```python
from build123d import *

# Parameters (mm, degrees)
SKETCH1_W               = 120
SKETCH1_H               = 85
BOSS_EXTRUDE1_DEPTH     = 17.5
SKETCH2_R               = 6.25
CUT_EXTRUDE1_DEPTH      = 34
SKETCH5_R               = 4
CUT_EXTRUDE4_DEPTH      = 82.432487375
FILLET1_R               = 5
SKETCH3_W               = 104.211367546
SKETCH3_H               = 27
CUT_EXTRUDE2_DEPTH      = 106.50473923
SKETCH4_W               = 69.558922102
SKETCH4_H               = 27
CUT_EXTRUDE3_DEPTH      = 129.500972759
SKETCH6_W               = 4
SKETCH6_H               = 4
BOSS_EXTRUDE2_DEPTH     = 35
CHAMFER1_SIZE           = 1
CHAMFER3_SIZE           = 1
CUT_EXTRUDE8_DEPTH      = 76.581082289
CUT_EXTRUDE8_DEPTH_BACK = 13.5
SKETCH10_W              = 127.378136422
SKETCH10_H              = 96.398058909
SKETCH11_W              = 4
SKETCH11_H              = 4
CUT_EXTRUDE9_DEPTH      = 82.432487375


with BuildPart() as part:
    # Sketch1 → Boss-Extrude1 (new, symmetric)
    with BuildSketch(Plane(origin=(0, 0, 0), x_dir=(1, 0, 0), z_dir=(0, 1, 0))):
        Rectangle(SKETCH1_W, SKETCH1_H)
    extrude(amount=BOSS_EXTRUDE1_DEPTH, both=True)

    # Sketch2 → Cut-Extrude1 (cut)
    with BuildSketch(Plane(origin=(0, 17.5, 0), x_dir=(1, 0, 0), z_dir=(0, 1, 0))):
        with Locations(Location((-45.56575, 27, 0), (0, 0, 270))):
            Circle(SKETCH2_R)
        with Locations(Location((-27.33945, 27, 0), (0, 0, 270))):
            Circle(SKETCH2_R)
        with Locations(Location((-9.11315, 27, 0), (0, 0, 270))):
            Circle(SKETCH2_R)
        with Locations(Location((9.11315, 27, 0), (0, 0, 270))):
            Circle(SKETCH2_R)
        with Locations(Location((27.33945, 27, 0), (0, 0, 270))):
            Circle(SKETCH2_R)
        with Locations(Location((45.56575, 27, 0), (0, 0, 270))):
            Circle(SKETCH2_R)
        with Locations(Location((-27.33945, 9, 0), (0, 0, 270))):
            Circle(SKETCH2_R)
        with Locations(Location((-9.11315, 9, 0), (0, 0, 270))):
            Circle(SKETCH2_R)
        with Locations(Location((9.11315, 9, 0), (0, 0, 270))):
            Circle(SKETCH2_R)
        with Locations(Location((27.33945, 9, 0), (0, 0, 270))):
            Circle(SKETCH2_R)
        with Locations(Location((45.56575, 9, 0), (0, 0, 270))):
            Circle(SKETCH2_R)
        with Locations(Location((-27.33945, -9, 0), (0, 0, 270))):
            Circle(SKETCH2_R)
        with Locations(Location((-9.11315, -9, 0), (0, 0, 270))):
            Circle(SKETCH2_R)
        with Locations(Location((9.11315, -9, 0), (0, 0, 270))):
            Circle(SKETCH2_R)
        with Locations(Location((27.33945, -9, 0), (0, 0, 270))):
            Circle(SKETCH2_R)
        with Locations(Location((45.56575, -9, 0), (0, 0, 270))):
            Circle(SKETCH2_R)
        with Locations(Location((-27.33945, -27, 0), (0, 0, 270))):
            Circle(SKETCH2_R)
        with Locations(Location((-9.11315, -27, 0), (0, 0, 270))):
            Circle(SKETCH2_R)
        with Locations(Location((9.11315, -27, 0), (0, 0, 270))):
            Circle(SKETCH2_R)
        with Locations(Location((27.33945, -27, 0), (0, 0, 270))):
            Circle(SKETCH2_R)
        with Locations(Location((45.56575, -27, 0), (0, 0, 270))):
            Circle(SKETCH2_R)
        with Locations(Location((-45.56575, 9, 0), (0, 0, 270))):
            Circle(SKETCH2_R)
        with Locations(Location((-45.56575, -9, 0), (0, 0, 270))):
            Circle(SKETCH2_R)
        with Locations(Location((-45.56575, -27, 0), (0, 0, 270))):
            Circle(SKETCH2_R)
    extrude(amount=-CUT_EXTRUDE1_DEPTH, mode=Mode.SUBTRACT)

    # Sketch5 → Cut-Extrude4 (cut, through all)
    with BuildSketch(Plane(origin=(0, 17.5, 0), x_dir=(1, 0, 0), z_dir=(0, 1, 0))):
        with Locations(Location((-45.56575, 27, 0), (0, 0, 270))):
            Circle(SKETCH5_R)
        with Locations(Location((-27.336055, 27, 0), (0, 0, 270))):
            Circle(SKETCH5_R)
        with Locations(Location((-9.10636, 27, 0), (0, 0, 270))):
            Circle(SKETCH5_R)
        with Locations(Location((9.123335, 27, 0), (0, 0, 270))):
            Circle(SKETCH5_R)
        with Locations(Location((27.35303, 27, 0), (0, 0, 270))):
            Circle(SKETCH5_R)
        with Locations(Location((45.582725, 27, 0), (0, 0, 270))):
            Circle(SKETCH5_R)
        with Locations(Location((-27.336055, 9, 0), (0, 0, 270))):
            Circle(SKETCH5_R)
        with Locations(Location((-9.10636, 9, 0), (0, 0, 270))):
            Circle(SKETCH5_R)
        with Locations(Location((9.123335, 9, 0), (0, 0, 270))):
            Circle(SKETCH5_R)
        with Locations(Location((27.35303, 9, 0), (0, 0, 270))):
            Circle(SKETCH5_R)
        with Locations(Location((45.582725, 9, 0), (0, 0, 270))):
            Circle(SKETCH5_R)
        with Locations(Location((-27.336055, -9, 0), (0, 0, 270))):
            Circle(SKETCH5_R)
        with Locations(Location((-9.10636, -9, 0), (0, 0, 270))):
            Circle(SKETCH5_R)
        with Locations(Location((9.123335, -9, 0), (0, 0, 270))):
            Circle(SKETCH5_R)
        with Locations(Location((27.35303, -9, 0), (0, 0, 270))):
            Circle(SKETCH5_R)
        with Locations(Location((45.582725, -9, 0), (0, 0, 270))):
            Circle(SKETCH5_R)
        with Locations(Location((-27.336055, -27, 0), (0, 0, 270))):
            Circle(SKETCH5_R)
        with Locations(Location((-9.10636, -27, 0), (0, 0, 270))):
            Circle(SKETCH5_R)
        with Locations(Location((9.123335, -27, 0), (0, 0, 270))):
            Circle(SKETCH5_R)
        with Locations(Location((27.35303, -27, 0), (0, 0, 270))):
            Circle(SKETCH5_R)
        with Locations(Location((45.582725, -27, 0), (0, 0, 270))):
            Circle(SKETCH5_R)
        with Locations(Location((-45.56575, 9, 0), (0, 0, 270))):
            Circle(SKETCH5_R)
        with Locations(Location((-45.56575, -9, 0), (0, 0, 270))):
            Circle(SKETCH5_R)
        with Locations(Location((-45.56575, -27, 0), (0, 0, 270))):
            Circle(SKETCH5_R)
    extrude(amount=-CUT_EXTRUDE4_DEPTH, mode=Mode.SUBTRACT)

    # Fillet1
    fillet1_edges = [part.edges().sort_by_distance(p)[0] for p in [
        (60, 0, 42.5),
        (-60, 0, 42.5),
        (-60, 0, -42.5),
        (60, 0, -42.5),
    ]]
    fillet(fillet1_edges, radius=FILLET1_R)

    # Sketch3 → Cut-Extrude2 (cut, through all)
    with BuildSketch(Plane(origin=(0, 0, -42.5), x_dir=(-1, 0, 0), z_dir=(0, 0, -1))):
        Rectangle(SKETCH3_W, SKETCH3_H)
    extrude(amount=-CUT_EXTRUDE2_DEPTH, mode=Mode.SUBTRACT)

    # Sketch4 → Cut-Extrude3 (cut, through all)
    with BuildSketch(Plane(origin=(60, 0, 0), x_dir=(0, 0, -1), z_dir=(1, 0, 0))):
        Rectangle(SKETCH4_W, SKETCH4_H)
    extrude(amount=-CUT_EXTRUDE3_DEPTH, mode=Mode.SUBTRACT)

    # Sketch6 → Boss-Extrude2 (add)
    with BuildSketch(Plane(origin=(0, 17.5, 0), x_dir=(1, 0, 0), z_dir=(0, 1, 0))):
        Rectangle(SKETCH6_W, SKETCH6_H)
    extrude(amount=-BOSS_EXTRUDE2_DEPTH)

    # Chamfer1
    chamfer1_edges = [part.edges().sort_by_distance(p)[0] for p in [
        (0, 13.5, -2),
        (-2, 13.5, 0),
        (0, 13.5, 2),
        (2, 13.5, 0),
        (2, -13.5, 0),
        (0, -13.5, 2),
        (-2, -13.5, 0),
        (0, -13.5, -2),
    ]]
    chamfer(chamfer1_edges, length=CHAMFER1_SIZE)

    # Chamfer3
    chamfer3_edges = [part.edges().sort_by_distance(p)[0] for p in [
        (-45.56575, 17.5, -33.25),
        (-27.33945, 17.5, -33.25),
        (-9.11315, 17.5, -33.25),
        (9.11315, 17.5, -33.25),
        (27.33945, 17.5, -33.25),
        (45.56575, 17.5, -33.25),
        (-27.33945, 17.5, -15.25),
        (-9.11315, 17.5, -15.25),
        (9.11315, 17.5, -15.25),
        (27.33945, 17.5, -15.25),
        (45.56575, 17.5, -15.25),
        (-27.33945, 17.5, 2.75),
        (-9.11315, 17.5, 2.75),
        (9.11315, 17.5, 2.75),
        (27.33945, 17.5, 2.75),
        (45.56575, 17.5, 2.75),
        (-27.33945, 17.5, 20.75),
        (-9.11315, 17.5, 20.75),
        (9.11315, 17.5, 20.75),
        (27.33945, 17.5, 20.75),
        (45.56575, 17.5, 20.75),
        (-45.56575, 17.5, -15.25),
        (-45.56575, 17.5, 2.75),
        (-45.56575, 17.5, 20.75),
    ]]
    chamfer(chamfer3_edges, length=CHAMFER3_SIZE)

    # Sketch10 → Cut-Extrude8 (cut, two sides: drawn at the far end of the back side and taken through both)
    with BuildSketch(Plane(origin=(0, 0, 0), x_dir=(1, 0, 0), z_dir=(0, 1, 0)).offset(-CUT_EXTRUDE8_DEPTH_BACK)):
        with Locations((-1.294046217, -0.232811032)):
            Rectangle(SKETCH10_W, SKETCH10_H)
    extrude(amount=CUT_EXTRUDE8_DEPTH + CUT_EXTRUDE8_DEPTH_BACK, mode=Mode.SUBTRACT)

    # Sketch11 → Cut-Extrude9 (cut, through all)
    with BuildSketch(Plane(origin=(0, 17.5, 0), x_dir=(1, 0, 0), z_dir=(0, 1, 0))):
        with Locations((-54.051771282, -36.924441912)):
            Rectangle(SKETCH11_W, SKETCH11_H)
        with Locations((53.948228718, -37.075558088)):
            Rectangle(SKETCH11_W, SKETCH11_H)
        with Locations((54.051771282, 36.924441912)):
            Rectangle(SKETCH11_W, SKETCH11_H)
        with Locations((-53.948228718, 37.075558088)):
            Rectangle(SKETCH11_W, SKETCH11_H)
        Rectangle(SKETCH11_W, SKETCH11_H)
    extrude(amount=-CUT_EXTRUDE9_DEPTH, mode=Mode.SUBTRACT)


solid = part.part
```
Geometry: final body of the model. Coordinates: model frame, mm. A direction names the side the tool comes from. Round coordinates to 2 decimals unless told otherwise and drop trailing zeros. Use CSV: the item, a comma, the result in double quotes. Start each with the question number.
Q1. Material intervals for line 1 along Z through (x, y) = (1, -15.05); line 2 along X through (y, z) = (-17.15, 1); line 3 along Z through (x, y) = (-41, -14.9), sorted ascending. Write a range as from..to.
Q2. Section query A-A (z = 27). State how many separate pieces and enclosed holes the cut face has, and give its area (3 significant figures).
Q3. First-contact query: pin 1 (11 mm diameter, centred on x = 45.57, z = 27, fed in from +Y); pin 2 (7 mm diameter, centred on x = 45.58, z = 9, fed in from -Y). Flat tips, straight axial feed; report the tip coordinate or a pass-through.
Q4. Access query for faces 3 (the face through (-50, -16.5, -9)), 4 (the face through (-52.052, -15, 37)). Directions: +Z, -Z, +X, -X, +Y, -Y. A direction counts if a zero-diameter tool reaches every point of the face in a straight line with its end or side. Return the directions, or none.
Q5. Mould query, pull axis X, two halves, no side actions, for faces 1 (the face through (-31.4, -16.5, 10.3)), 2 (the face through (-58.57, -15.47, 41)). Classes: +X half, -X half, draft (parallel to the pull), parting line (faces both ways), or undercut.
Result set:
1,line 1,"z = -42.5..-2, 2..42.5"
1,line 2,"x = -60..-2, 2..60"
1,line 3,"z = -42.5..-31.27, -22.73..-13.27, -4.73..4.73, 13.27..22.73, 31.27..42.5"
2,separate pieces,"7"
2,enclosed holes,"0"
2,area,"207 mm2"
3,pin 1,"stops at y = -16.5"
3,pin 2,"passes through"
4,face 3,"+Y"
4,face 4,"+Y, -Y"
5,face 1,"undercut"
5,face 2,"-X half"
